Input: dimensioned drawing with shaded views. Units: mm. Origin: part minimum x, y, z. A direction names the side the tool comes from. Round coordinates to 2 decimals unless told otherwise and drop trailing zeros. Loops run counter-clockwise (first coordinate to the right, second up) from the corner with the lowest first, then second, coordinate; pieces in that order, holes last. Notation, with made-up numbers: (-18.5, -18) - (16.5, -18) arc R22 ccw to (16.5, 16) - close; hole circle Ø8 at (79, 66.25). An arc over 180 degrees is marked (long way). One line per question, with ' | ' between items. Start each with the question number.
Item 1: Section B-B, the plane z = 6. Return loops of the section in (x, y), plus the area to 3 significant figures.
Item 2: Section D-D, the plane x = 63.5. Return loops of the section in (y, z).
Item 3: Section C-C, the plane y = 43. Return loops of the section in (x, z).
Item 4: Set-up query: the marked faces 1, 2, 3, 4 and 5. Return all of +Z, -Z, +X, -X, +Y, -Y with unobstructed straight access to the full face (end or side cutting, diameter ignored); none if empty.
Item 5: First-contact query: pin 1 (9.5 mm diameter, centred on y = 46, z = 5, fed in from +X). Flat tip, straight axial feed; report the tip coordinate or a pass-through.
Item 6: Draft query along X for the marked faces 6, 7, 8 and 9. Return one class per face: pulls with the +X half, pulls with the -X half, needs draft (parallel to the pull), parting line crosses it, or undercut.
Item 7: Section A-A, the plane x = 115.5. Return loops of the section in (y, z).
Item 8: Material intervals for line 1 along X through (y, z) = (21, 13); line 2 along Z through (x, y) = (60.5, 51); line 3 along X through (y, z) = (14.5, 36), sorted ascending.
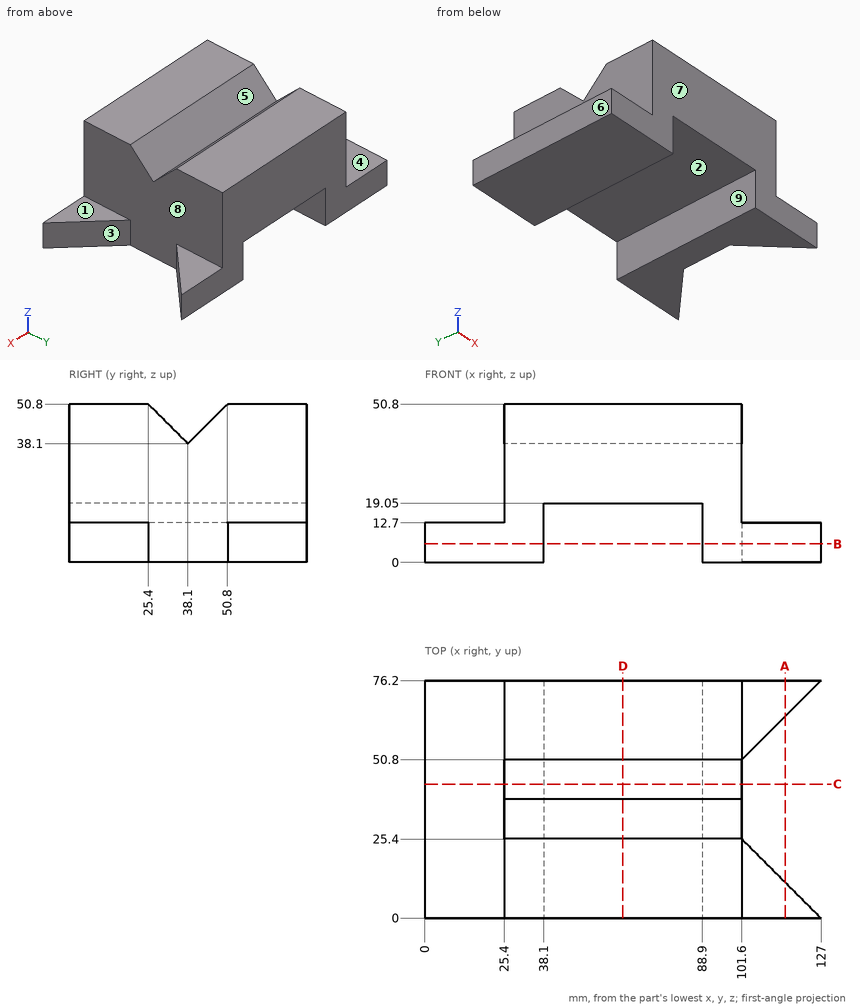
Return value:
1) outline: (0, 0) - (38.1, 0) - (38.1, 76.2) - (0, 76.2) - close; (88.9, 0) - (127, 0) - (101.6, 25.4) - (101.6, 50.8) - (127, 76.2) - (88.9, 76.2) - close | area: 4,520 mm2
2) outline: (0, 19.05) - (76.2, 19.05) - (76.2, 50.8) - (50.8, 50.8) - (38.1, 38.1) - (25.4, 50.8) - (0, 50.8) - close
3) outline: (0, 0) - (38.1, 0) - (38.1, 19.05) - (88.9, 19.05) - (88.9, 0) - (101.6, 0) - (101.6, 43) - (25.4, 43) - (25.4, 12.7) - (0, 12.7) - close
4) face 1: +Z, +X, +Y, -Y | face 2: -Z, +Y, -Y | face 3: +Z, -Z, +X | face 4: +Z, -X, +Y, -Y | face 5: +Z, +X, -X
5) pin 1: x = 101.6
6) face 6: pulls with the -X half | face 7: needs draft | face 8: pulls with the +X half | face 9: undercut
7) outline: (0, 0) - (11.5, 0) - (11.5, 12.7) - (0, 12.7) - close; (64.7, 0) - (76.2, 0) - (76.2, 12.7) - (64.7, 12.7) - close
8) line 1: 25.4 to 38.1, 88.9 to 101.6 | line 2: 19.05 to 50.8 | line 3: 25.4 to 101.6
